The model under review builds one solid part; all positions refer to its coordinate system, in mm. Face numbers are marked on the shaded views. A direction names the side the tool comes from. Coordinates: 2 decimals unless noted, no trailing zeros. Write each loop counter-clockwise with the first axis right and the second up, starting at its lowest first coordinate (ties: lowest second). Pieces come first, ordered by that corner, then holes.
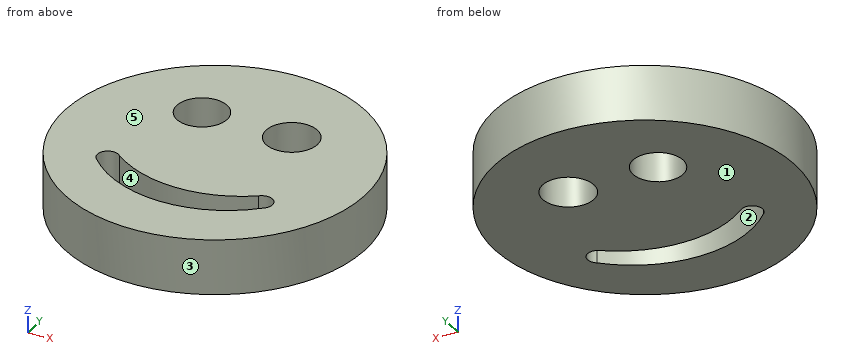
```python
from build123d import *

# Parameters (mm, degrees)
F0_R     = 68.746685
F0_R_2   = 11.512812
F0_R_3   = 11.746204
F1_DEPTH = 25.4


with BuildPart() as f1:
    # F0 (on Top) → F1 (new body)
    with BuildSketch(Plane.XY):
        Circle(F0_R)
        with BuildLine():
            ThreePointArc((38.200267, -28.575001), (-0.489346, -44.214171), (-38.801841, -27.672632))
            ThreePointArc((-38.801841, -27.672632), (-38.972847, -20.885155), (-32.184474, -20.754473))
            ThreePointArc((-32.184474, -20.754473), (-0.200583, -31.594777), (31.883683, -21.055264))
            ThreePointArc((31.883683, -21.055264), (39.13117, -21.380206), (38.200267, -28.575001))
        make_face(mode=Mode.SUBTRACT)
        with Locations((-20.152895, 24.965527)):
            Circle(F0_R_2, mode=Mode.SUBTRACT)
        with Locations((20.754473, 25.567105)):
            Circle(F0_R_3, mode=Mode.SUBTRACT)
    extrude(amount=F1_DEPTH)


solid = f1.part
```
Item 1: Machinability: for the marked faces 1 and 2, which of the approach directions +Z, -Z, +X, -X, +Y, -Y give a long, thin tool a straight path to every point of the face, cutting with its end or side? Answer none if there is none.
Solved:
face 1: -Z, +X, -X, +Y, -Y
face 2: +Z, -Z
Item 2: Mouldability with a two-part tool opening along Y and no side actions: class the marked faces 3, 4 and 5 as pulls with the +Y half, pulls with the -Y half, needs draft (parallel to the pull), parting line crosses it, or undercut.
Solved:
face 3: parting line crosses it
face 4: undercut
face 5: needs draft
Item 3: Take a section at B-B, the plane z = 18.25. Write out the cut boundary in (x, y) (1 decimal), plus the area to 3 significant figures.
Solved:
outline: circle Ø137.5 at (0, 0); hole (-38.8, -27.7) arc R54.1 ccw to (38.2, -28.6) arc R4.9 ccw (long way) to (31.9, -21.1) arc R53.3 cw to (-32.2, -20.8) arc R4.8 ccw (long way) to start; hole circle Ø23 at (-20.2, 25); hole circle Ø23.5 at (20.8, 25.6)
area: 13,000 mm2
Item 4: For pin 1 (2 mm diameter, centred on x = 44.5, z = 12, fed in from +Y); pin 2 (8 mm diameter, centred on x = 35.36, y = -24.55, fed in from +Z) (3 decimals); pin 3 (2 mm diameter, centred on y = 10.5, z = 10, fed in from -X); pin 4 (12 mm diameter, centred on y = 38, z = 19, fed in from -X), all flat-tipped, find the tip position at first contact; note any pin that passes through.
Solved:
pin 1: stops at y = 53.23
pin 2: passes through
pin 3: stops at x = -68.09
pin 4: stops at x = -60.84
Item 5: To check wall thickness, follow line 1 along Y through (x, z) = (-10.5, 3.25); line 2 along X through (y, z) = (32, 8.5); line 3 along X through (y, z) = (18, 11). State the ranges of each line that lie inside material, in increasing order.
Solved:
line 1: y = -67.94 to -43.16, -30.54 to 18.69, 31.24 to 67.94
line 2: x = -60.84 to -29.27, -11.04 to 10.93, 30.58 to 60.84
line 3: x = -66.35 to -29.32, -10.99 to 11.77, 29.74 to 66.35
Item 6: Take a section at A-A, the plane x = 0. Write out the cut boundary in (y, z), plus the area to 3 significant figures.
Solved:
outline: (-68.75, 0) - (-44.22, 0) - (-44.22, 25.4) - (-68.75, 25.4) - close; (-31.6, 0) - (68.75, 0) - (68.75, 25.4) - (-31.6, 25.4) - close
area: 3,170 mm2
Item 7: Take a section at C-C, the plane y = -42. Write out the cut boundary in (x, z).
Solved:
outline: (-54.43, 0) - (-15.19, 0) - (-15.19, 25.4) - (-54.43, 25.4) - close; (15.48, 0) - (54.43, 0) - (54.43, 25.4) - (15.48, 25.4) - close
Item 8: Take a section at D-D, the plane y = -13. Write out the cut boundary in (x, z), plus the area to 3 significant figures.
Solved:
outline: (-67.51, 0) - (67.51, 0) - (67.51, 25.4) - (-67.51, 25.4) - close
area: 3,430 mm2
